from build123d import *

# Parameters (mm, degrees)
SKETCH1_R            = 1.75
BOSS_EXTRUDE1_DEPTH  = 3.175
SHELL1_START         = -13.3528
SHELL1_OUTLINE_W     = 3.5306
SHELL1_OUTLINE_H     = 6.35
SHELL1_DEPTH         = 0.1778
SHELL1_START_2       = -6.825
SHELL1_2_OUTLINE_W   = 3.5306
SHELL1_2_OUTLINE_H   = 6.35
SHELL1_2_DEPTH       = 0.1778
SHELL1_START_3       = -20.1778
SHELL1_3_OUTLINE_W   = 3.5306
SHELL1_3_OUTLINE_H   = 25.3075948
SHELL1_3_DEPTH       = 20.3556
SHELL1_START_4       = -13.175
SHELL1_4_OUTLINE_W   = 3.5306
SHELL1_4_OUTLINE_H   = 6.35
SHELL1_4_DEPTH       = 6.35
SHELL1_5_OUTLINE_R   = 1.75
SHELL1_5_OUTLINE_R_2 = 1.5722
SHELL1_5_DEPTH       = 3.175
SHELL1_START_5       = -0.1778
SHELL1_6_OUTLINE_R   = 1.5722
SHELL1_6_DEPTH       = 3.5306


with BuildPart() as part:
    # Sketch1 → Boss-Extrude1 (new body)
    with BuildSketch(Plane(origin=(0, 0, 0), x_dir=(0, 0, -1), z_dir=(1, 0, 0))):
        Polygon((0, 0), (6.825, 0), (6.825, -6.35), (13.175, -6.35), (13.175, 0), (20, 0), (20, 6.629574014), (14.471500996, 10.288392178), (14.471500996, 14.663602622), (20, 18.322420786), (20, 24.9519948), (0, 24.9519948), (0, 18.322420786), (5.528499004, 14.663602622), (5.528499004, 10.288392178), (0, 6.629574014), align=None)
        with Locations((10, 19.9519948)):
            Circle(SKETCH1_R, mode=Mode.SUBTRACT)
        with Locations((10, 2.4259948)):
            Circle(SKETCH1_R, mode=Mode.SUBTRACT)
    extrude(amount=BOSS_EXTRUDE1_DEPTH)

    # Shell1: read off the stored shape, not the designer's step
    # Shell1 outline → Shell1 (add)
    with BuildSketch(Plane.XY.offset(SHELL1_START)):
        with Locations((1.5875, -3.3528)):
            Rectangle(SHELL1_OUTLINE_W, SHELL1_OUTLINE_H)
    extrude(amount=SHELL1_DEPTH)

    # Shell1 2 outline → Shell1 2 (add)
    with BuildSketch(Plane.XY.offset(SHELL1_START_2)):
        with Locations((1.5875, -3.3528)):
            Rectangle(SHELL1_2_OUTLINE_W, SHELL1_2_OUTLINE_H)
    extrude(amount=SHELL1_2_DEPTH)

    # Shell1 3 outline → Shell1 3 (add)
    with BuildSketch(Plane.XY.offset(SHELL1_START_3)):
        with Locations((1.5875, 12.4759974)):
            Rectangle(SHELL1_3_OUTLINE_W, SHELL1_3_OUTLINE_H)
    extrude(amount=SHELL1_3_DEPTH)

    # Shell1 4 outline → Shell1 4 (add)
    with BuildSketch(Plane.XY.offset(SHELL1_START_4)):
        with Locations((1.5875, -3.3528)):
            Rectangle(SHELL1_4_OUTLINE_W, SHELL1_4_OUTLINE_H)
    extrude(amount=SHELL1_4_DEPTH)

    # Shell1 5 outline → Shell1 5 (cut)
    # profile 1 of 5: a face of its own
    with BuildSketch(Plane.YZ):
        Polygon((14.568061248, -14.649300996), (10.383933552, -14.649300996), (6.725115387, -20.1778), (18.226879413, -20.1778), align=None)
    # profile 2 of 5: a face of its own
    with BuildSketch(Plane.YZ):
        Polygon((10.383933552, -5.350699004), (14.568061248, -5.350699004), (18.226879413, 0.1778), (6.725115387, 0.1778), align=None)
    # profile 3 of 5: a face of its own
    with BuildSketch(Plane.YZ):
        Polygon((6.629574014, 0), (0, 0), (0, -6.825), (-6.35, -6.825), (-6.35, -13.175), (0, -13.175), (0, -20), (6.629574014, -20), (10.288392178, -14.471500996), (14.663602622, -14.471500996), (18.322420786, -20), (24.9519948, -20), (24.9519948, 0), (18.322420786, 0), (14.663602622, -5.528499004), (10.288392178, -5.528499004), align=None)
        with Locations((2.4259948, -10)):
            Circle(SHELL1_5_OUTLINE_R, mode=Mode.SUBTRACT)
        with Locations((19.9519948, -10)):
            Circle(SHELL1_5_OUTLINE_R, mode=Mode.SUBTRACT)
    # profile 4 of 5: a face of its own
    with BuildSketch(Plane.YZ):
        with Locations((2.4259948, -10)):
            Circle(SHELL1_5_OUTLINE_R_2)
    # profile 5 of 5: a face of its own
    with BuildSketch(Plane.YZ):
        with Locations((19.9519948, -10)):
            Circle(SHELL1_5_OUTLINE_R_2)
    extrude(amount=SHELL1_5_DEPTH, mode=Mode.SUBTRACT)

    # Shell1 6 outline → Shell1 6 (cut)
    with BuildSketch(Plane.YZ.offset(SHELL1_START_5)):
        Polygon((14.568061248, -14.649300996), (10.383933552, -14.649300996), (6.725115387, -20.1778), (18.226879413, -20.1778), align=None)
        Polygon((10.383933552, -5.350699004), (14.568061248, -5.350699004), (18.226879413, 0.1778), (6.725115387, 0.1778), align=None)
        with Locations((19.9519948, -10)):
            Circle(SHELL1_6_OUTLINE_R)
        with Locations((2.4259948, -10)):
            Circle(SHELL1_6_OUTLINE_R)
    extrude(amount=SHELL1_6_DEPTH, mode=Mode.SUBTRACT)


solid = part.part
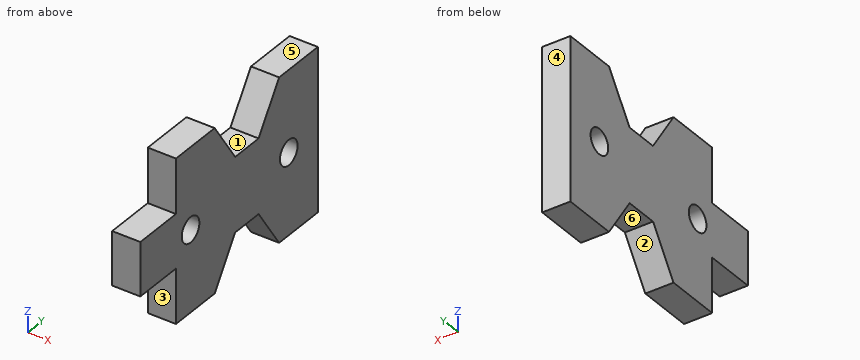
Model file for the job. Use its own axes, mm. Face numbers are marked on the shaded views. A direction names the side the tool comes from. Round coordinates to 2 decimals unless told otherwise and drop trailing zeros. Order: outer loops, then holes, each group sorted by start corner. A loop starts at its lowest first (then second) coordinate and runs counter-clockwise, first axis right, second up.
(1) Band-saw the part on B-B (x = 2.75). Give the number of separate pieces and of enclosed holes in the cut face, then the cut area to 3 significant figures.
(2) Drill centre lines: line 1 (Z direction, x = 2.3, y = 1); line 2 (Y direction, x = 0.35, z = -14); line 3 (X direction, y = 15, z = -14) (3 decimals). Where is each one in solid material? Low to high.
(3) Band-saw the part on A-A (z = -10). List the corners of the cut face in (x, y) (3 decimals), then the cut area to 3 significant figures.
(4) Band-saw the part on C-C (y = 17). List the corners of the cut face in (x, z) (3 decimals), then the cut area to 3 significant figures.
(5) Pin check, flat tips, straight feed: pin 1 (1.1 mm diameter, centred on x = 1.5, y = 12, fed in from -Z); pin 2 (1.5 mm diameter, centred on y = -2, z = -17.5, fed in from +X); pin 3 (1.1 mm diameter, centred on x = 2.5, y = -4.5, fed in from +Z); pin 4 (1.1 mm diameter, centred on x = 2.5, y = -4, fed in from -Z). Stop position of each tip, or through.
(6) 3-axis set-ups, long thin cutter, end or side, ignore diameter. For the marked faces 1, 2 and 3: which of +Z, -Z, +X, -X, +Y, -Y reach the whole face in a straight line?
(7) Pull direction Y, two halves, no side cores. Call the marked faces 4, 5 and 6: released by +Y, released by -Y, zero draft, split by the parting line, or undercut.
Verdict:
1. separate pieces: 3
1. enclosed holes: 3
1. area: 24.2 mm2
2. line 1: z = -20.18 to -20, -11.01 to -10.66, -9.34 to -8.99, 0 to 0.18
2. line 2: y = -0.18 to 0, 24.95 to 25.13
2. line 3: x = -0.178 to 0, 3.175 to 3.353
3. outline: (-0.178, -6.528) - (3.353, -6.528) - (3.353, 0.854) - (-0.178, 0.854) - close; (-0.178, 3.998) - (3.353, 3.998) - (3.353, 18.38) - (-0.178, 18.38) - close; (-0.178, 21.524) - (3.353, 21.524) - (3.353, 25.13) - (-0.178, 25.13) - close; hole (0, -6.35) - (3.175, -6.35) - (3.175, 0.676) - (0, 0.676) - close; hole (0, 4.176) - (3.175, 4.176) - (3.175, 18.202) - (0, 18.202) - close; hole (0, 21.702) - (3.175, 21.702) - (3.175, 24.952) - (0, 24.952) - close
3. area: 12.4 mm2
4. outline: (-0.178, -18.324) - (3.353, -18.324) - (3.353, -1.676) - (-0.178, -1.676) - close; hole (0, -18.002) - (3.175, -18.002) - (3.175, -1.998) - (0, -1.998) - close
4. area: 7.97 mm2
5. pin 1: stops at z = -14.65
5. pin 2: passes through
5. pin 3: stops at z = -6.65
5. pin 4: stops at z = -13.35
6. face 1: +Z, +X, -X
6. face 2: -Z, +X, -X
6. face 3: -Z, +X, -X, -Y
7. face 4: released by +Y
7. face 5: zero draft
7. face 6: undercut
